```python
from build123d import *

# Parameters (mm, degrees)
BOSS_EXTRUDE1_DEPTH = 10
CHAMFER1_SIZE       = 0.5
SKETCH7_W           = 1
SKETCH7_H           = 3
SKETCH7_H_2         = 1
CUT_EXTRUDE1_DEPTH  = 14.310211959


with BuildPart() as part:
    # Sketch2 → Boss-Extrude1 (new body)
    with BuildSketch(Plane.XY):
        Polygon((4.25, 0), (5.75, 0), (5.75, -2.5), (4.335786438, -3.914213562), (5.042893219, -4.621320344), (6.75, -2.914213562), (6.75, 1), (0, 1), (0, 0), (3.45, 0), (3.45, -0.4), (3.65, -0.4), (3.65, -0.5), (4.05, -0.5), (4.05, -0.4), (4.25, -0.4), align=None)
    boss_extrude1 = extrude(amount=BOSS_EXTRUDE1_DEPTH)

    # Mirror1: Boss-Extrude1 across plane
    add(boss_extrude1.mirror(Plane(origin=(0, 0, 0), x_dir=(0, 0, 1), z_dir=(1, 0, 0))))

    # Chamfer1
    chamfer1_edges = [part.edges().sort_by_distance(p)[0] for p in [
        (6.75, 1, 5),
        (-6.75, 1, 5),
    ]]
    chamfer(chamfer1_edges, length=CHAMFER1_SIZE)

    # Sketch7 → Cut-Extrude1 (cut, through all)
    with BuildSketch(Plane(origin=(0, 1, 0), x_dir=(1, 0, 0), z_dir=(0, 1, 0))):
        with Locations((0, -5)):
            Rectangle(SKETCH7_W, SKETCH7_H)
        with Locations((0, -3)):
            Rectangle(SKETCH7_W, SKETCH7_H_2)
        with Locations((0, -7)):
            Rectangle(SKETCH7_W, SKETCH7_H_2)
        with Locations((2, -5)):
            Rectangle(SKETCH7_W, SKETCH7_H)
        with Locations((-2, -5)):
            Rectangle(SKETCH7_W, SKETCH7_H)
    extrude(amount=-CUT_EXTRUDE1_DEPTH, mode=Mode.SUBTRACT)


solid = part.part
```
Can you work these out from the model? Positions are in its coordinate system, mm. A direction names the side the tool comes from. Round coordinates to 2 decimals unless told otherwise and drop trailing zeros. Loops run counter-clockwise (first coordinate to the right, second up) from the corner with the lowest first, then second, coordinate; pieces in that order, holes last. Notation, with made-up numbers: M 85.5,82 L 124.5,82 A15 cw 124.5,96 Z; hole C 17,-14 d10. An arc over 180 degrees is marked long. Answer as a JSON object with one key per item and string values. Group by question number.
Q1. Imagine slicing it at C-C, the plane x = -1.75. Please give me the cut outline in (y, z).
Q2. Please list where these lines run through material, in increasing order: L1, parallel to X at y = -0.45, z = 3.5; L2, parallel to X at y = -1.5, z = 8.5; L3, parallel to Y at x = -2.75, z = 3.5.
Q3. We'd pull the mould along Y, two halves only. Please class faces 1 (the flat face through (-2, 0.5, 6.5)), 2 (the flat face through (-1, 0, 5)), 3 (the flat face through (5.75, -1, 5)), 4 (the flat face through (-5.75, -1, 5)): +Y half, -Y half, draft (parallel to the pull), parting line (faces both ways), or undercut.
Q4. Imagine slicing it at B-B, the plane y = -1.45. Please give me the cut outline in (x, z), then the cut area to 3 significant figures.
Q5. Will this pin go through, and if not, where does the flat tip stop? pin 1 (3.5 mm diameter, centred on x = 1.5, z = 7, fed in from -Y).
Q6. On a 3-axis mill with a long thin cutter (end or side, diameter ignored), from which of +Z, -Z, +X, -X, +Y, -Y can I reach the whole of each face in a straight line? I mean faces 5 (the flat face through (-5, 0, 5)), 6 (the flat face through (-1.5, 0.5, 5)), 7 (the flat face through (6.75, -1, 5)). Say none if no direction works.
Findings:
{
 "1": {"outline": "M 0,0 L 1,0 L 1,3.5 L 0,3.5 Z; M 0,6.5 L 1,6.5 L 1,10 L 0,10 Z"},
 "2": {"L1": "x = -6.75 to -5.75, -4.05 to -3.65, 3.65 to 4.05, 5.75 to 6.75", "L2": "x = -6.75 to -5.75, 5.75 to 6.75", "L3": "y = 0 to 1"},
 "3": {"face 1": "draft", "face 2": "-Y half", "face 3": "undercut", "face 4": "undercut"},
 "4": {"outline": "M -6.75,0 L -5.75,0 L -5.75,10 L -6.75,10 Z; M 5.75,0 L 6.75,0 L 6.75,10 L 5.75,10 Z", "area": "20.0 mm2"},
 "5": {"pin 1": "stops at y = 0"},
 "6": {"face 5": "+Z, -Z", "face 6": "+Y, -Y", "face 7": "+Z, -Z, +X, +Y, -Y"}
}
